from build123d import *

# Parameters (mm, degrees)
SKETCH_1_W                     = 80
SKETCH_1_H                     = 37
EXTRUDE_1_DEPTH                = 27
SKETCH_2_W                     = 7
SKETCH_2_H                     = 6
CUT_EXTRUDE_1_DEPTH            = 61.811183182
PATTERN_LINEAR_1_COUNT         = 7
PATTERN_LINEAR_1_PITCH         = 7.8
SKETCH_3_W                     = 1.5
SKETCH_3_H                     = 15.5
HOLE_WIZARD_3_0_3_1_AT_2_COUNT = 2
HOLE_WIZARD_3_0_3_1_AT_2_PITCH = 16
HOLE_WIZARD_3_0_3_1_AT_3_COUNT = 2
HOLE_WIZARD_3_0_3_1_AT_3_PITCH = 32
HOLE_WIZARD_6_5_6_5_1_D        = 6.5
HOLE_WIZARD_3_0_3_2_D          = 3


with BuildPart() as part:
    # Эскиз1 → Бобышка-Вытянуть1 (new body)
    with BuildSketch(Plane(origin=(0, 0, 0), x_dir=(-1, 0, 0), z_dir=(0, 0, -1))):
        with Locations((0, -18.5)):
            Rectangle(SKETCH_1_W, SKETCH_1_H)
    extrude(amount=-EXTRUDE_1_DEPTH)

    # Эскиз2 → Вырез-Вытянуть1 (cut, through all)
    with BuildSketch(Plane.XZ.offset(37)):
        with Locations((-23.3, 8.5)):
            Rectangle(SKETCH_2_W, SKETCH_2_H)
    cut_extrude_1 = extrude(amount=-CUT_EXTRUDE_1_DEPTH, mode=Mode.SUBTRACT)

    # Линейный массив1: Вырез-Вытянуть1 ×7
    with Locations(*[(i * PATTERN_LINEAR_1_PITCH, 0, 0) for i in range(1, PATTERN_LINEAR_1_COUNT)]):
        add(cut_extrude_1, mode=Mode.SUBTRACT)

    # Эскиз3 → Диаметр отверстия Ø3.0 (3)1 (revolve, cut)
    with BuildSketch(Plane(origin=(16, -16, 11.5), x_dir=(0, 1, 0), z_dir=(1, 0, 0))):
        with Locations((0.75, 7.75)):
            Rectangle(SKETCH_3_W, SKETCH_3_H)
    hole_wizard_3_0_3_1 = revolve(axis=Axis((16, -16, 5.15), (0, 0, 1)), mode=Mode.SUBTRACT)

    # Диаметр отверстия Ø3.0 (3)1 at 2: Диаметр отверстия Ø3.0 (3)1 ×2
    with Locations(*[(-i * HOLE_WIZARD_3_0_3_1_AT_2_PITCH, 0, 0) for i in range(1, HOLE_WIZARD_3_0_3_1_AT_2_COUNT)]):
        add(hole_wizard_3_0_3_1, mode=Mode.SUBTRACT)

    # Диаметр отверстия Ø3.0 (3)1 at 3: Диаметр отверстия Ø3.0 (3)1 ×2
    with Locations(*[(-i * HOLE_WIZARD_3_0_3_1_AT_3_PITCH, 0, 0) for i in range(1, HOLE_WIZARD_3_0_3_1_AT_3_COUNT)]):
        add(hole_wizard_3_0_3_1, mode=Mode.SUBTRACT)

    # Диаметр отверстия Ø6.5 (6.5)1 (through all)
    with Locations(Plane(origin=(0, -37, 0), x_dir=(-1, 0, 0), z_dir=(0, -1, 0))):
        with Locations((30.75, -8.75), (-30.75, -8.75)):
            Hole(HOLE_WIZARD_6_5_6_5_1_D / 2)

    # Диаметр отверстия Ø3.0 (3)2 (through all)
    with Locations(Plane.XY.offset(5.5)):
        with Locations((16, -16), (0, -16), (-16, -16)):
            Hole(HOLE_WIZARD_3_0_3_2_D / 2)


solid = part.part
Can you work these out from the model? Positions are in its coordinate system, mm. A direction names the side the tool comes from. Coordinates: 2 decimals unless noted, no trailing zeros. Loops run counter-clockwise (first coordinate to the right, second up) from the corner with the lowest first, then second, coordinate; pieces in that order, holes last. Notation, with made-up numbers: (13.5, 23) - (19.5, 23) arc R31 cw to (19.5, 48) - close; hole circle Ø5 at (56, 34). An arc over 180 degrees is marked (long way). Answer as a JSON object with one key per item and string values. Group by question number.
Item 1: For pin 1 (2.5 mm diameter, centred on x = 0, y = -16, fed in from -Z), with a flat end and sliding along its axis, tell me the tip position at first contact or that it passes through.
Item 2: If I drill on L1, parallel to X at y = -16, z = 18.5; L2, parallel to Z at x = 21, y = -33.5; L3, parallel to Y at x = 0, z = 17, over which ranges is the centre line in solid material (lowest first)? Write a range as from..to.
Item 3: On a 3-axis mill with a long thin cutter (end or side, diameter ignored), from which of +Z, -Z, +X, -X, +Y, -Y can I reach the whole of each face in a straight line? I mean faces 1 (the face through (15.93, -17.5, 19.36)), 2 (the face through (23, -19, 11.5)). Say none if no direction works.
Item 4: If we section it at A-A (x = 16): List the corners of the cut face in (y, z) for me, plus the area to 3 significant figures.
Item 5: If we mould it in two halves opening along X, with no side actions, what happens to faces 3 (the face through (1, -18, 0)), 4 (the face through (-14.5, -15.93, 2.71))? For each: released by +X, released by -X, zero draft, split by the parting line, or undercut.
Item 6: If we section it at B-B (y = -9.5): State how many separate pieces and enclosed holes the cut face has, plus the area to 3 significant figures.
Returned:
{
 "1": {"pin 1": "passes through"},
 "2": {"L1": "x = -40..-17.5, -14.5..-1.5, 1.5..14.5, 17.5..40", "L2": "z = 0..5.5, 11.5..27", "L3": "y = -37..-17.5, -14.5..0"},
 "3": {"face 1": "+Z, -Z", "face 2": "+Y, -Y"},
 "4": {"outline": "(-37, 0) - (-17.5, 0) - (-17.5, 5.5) - (-37, 5.5) - close; (-37, 11.5) - (-17.5, 11.5) - (-17.5, 27) - (-37, 27) - close; (-14.5, 0) - (0, 0) - (0, 5.5) - (-14.5, 5.5) - close; (-14.5, 11.5) - (0, 11.5) - (0, 27) - (-14.5, 27) - close", "area": "714 mm²"},
 "5": {"face 3": "zero draft", "face 4": "undercut"},
 "6": {"separate pieces": "1", "enclosed holes": "9", "area": "1,800 mm²"}
}
